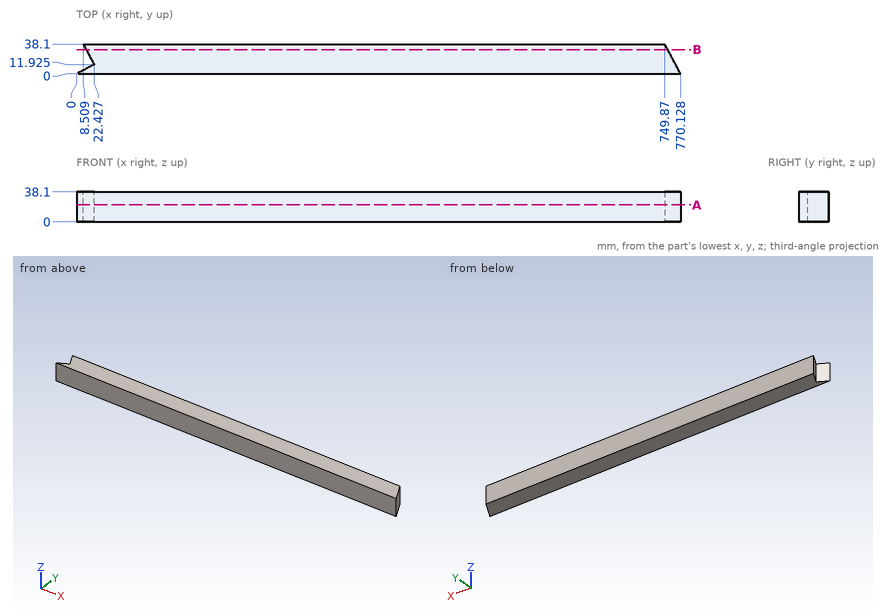
Answer from the drawing. Dimensions are ordinates in mm from the lowest x, y and z of the part. Give positions to 0.01 mm unless a question says otherwise; leave off trailing zeros. Loops run counter-clockwise (first coordinate to the right, second up) from the corner with the lowest first, then second, coordinate; pieces in that order, holes last.
Item 1: The part is cut by section A-A (z = 21.5). Write down the section's boundary in (x, y) (1 decimal), and give its area (3 significant figures).
Item 2: Find the intervals of material crossed by line 1 along X through (y, z) = (7.5, 28.5) (1 decimal); line 2 along X through (y, z) = (29, 8), in increasing order.
Item 3: The part is cut by section B-B (y = 31). Write down the section's boundary in (x, z) (1 decimal), and give its area (3 significant figures).
Item 4: Each of these flat-tipped pins is pushed along its axis until it touches: pin 1 Ø5 at (y, z) = (29.5, 6) entering from -X; pin 2 Ø1 at (y, z) = (26, 22) entering from +X; pin 3 Ø3 at (y, z) = (12, 34) entering from +X (1 decimal). Where does it stop, or does it pass through?
Taken from the geometry:
1. outline: (0, 0) - (770.1, 0) - (749.9, 38.1) - (8.5, 38.1) - (22.4, 11.9) - close
1. area: 28,400 mm2
2. line 1: x = 14.1 to 766.1
2. line 2: x = 13.35 to 754.71
3. outline: (12.3, 0) - (753.6, 0) - (753.6, 38.1) - (12.3, 38.1) - close
3. area: 28,200 mm2
4. pin 1: stops at x = 11.75
4. pin 2: stops at x = 756.57
4. pin 3: stops at x = 764.5
